Part model, mm, in its own coordinate system. Face numbers are marked on the shaded views. Give positions to 0.01 mm unless a question says otherwise; leave off trailing zeros. Write each loop counter-clockwise with the first axis right and the second up, starting at its lowest first coordinate (ties: lowest second). Pieces come first, ordered by that corner, then holes. Notation, with made-up numbers: M -4.5,57.5 L 50.5,57.5 A18 cw 50.5,91.5 Z; hole C 24,15.25 d6. An arc over 180 degrees is marked long. Answer as CSV lines item,"result". Start each with the question number.
1) Pin check, flat tips, straight feed: pin 1 Ø2 at (x, z) = (3, 7.5) entering from +Y; pin 2 Ø1 at (x, y) = (1, -22.5) entering from -Z; pin 3 Ø1.5 at (x, z) = (2, 13) entering from -Y. Stop position of each tip, or through.
2) Mould opens along Z. For the marked faces 1, 2 and 3 say: pulls with the +Z half, pulls with the -Z half, needs draft (parallel to the pull), parting line crosses it, or undercut.
3) Slice it at B-B, the plane y = -25.5. Give the cut face in (x, z).
4) Slice it at A-A, the plane x = 0.65. Give the cut face in (y, z), plus the area to 3 significant figures.
5) Wall check: line 1 along Z through (x, y) = (0.45, -21.75); line 2 along Y through (x, z) = (2.05, 10.25); line 3 along Y through (x, z) = (2.8, 10.75). Give the ranges that are in metal, low to high. Write a range as from..to.
6) Slice it at D-D, the plane x = 2.7. Give the cut face in (y, z), plus the area to 3 significant figures.
7) Slice it at C-C, the plane z = 6.25. Give the cut face in (x, y), plus the area to 3 significant figures.
```python
from build123d import *

# Parameters (mm, degrees)
SKETCH_1_R      = 5
EXTRUDE_1_DEPTH = 4
CHAMFER_1_SIZE  = 1.5
CHAMFER_1_SIZE2 = 1.616714541


with BuildPart() as part:
    # 草图1 → 凸台-拉伸1 (new body)
    with BuildSketch(Plane(origin=(0, 0, 0), x_dir=(0, 0, -1), z_dir=(1, 0, 0))):
        with Locations((-9.325362428, -21.699923803)):
            Circle(SKETCH_1_R)
    extrude(amount=EXTRUDE_1_DEPTH)

    # 切除-拉伸1 cone 1 section (through the dimple's axis) → 切除-拉伸1 (revolve, cut)
    with BuildSketch(Plane(origin=(4, -21.699923803, 9.325362428), x_dir=(0, 0, -1), z_dir=(0, 1, 0))):
        Polygon((0, 0), (1.3, 0), (0, 18.590866134), align=None)
    revolve(axis=Axis((4, -21.699923803, 9.325362428), (-1, 0, 0)), mode=Mode.SUBTRACT)

    # 倒角1
    chamfer_1_edges = [part.edges().sort_by_distance(p)[0] for p in [
        (4, -21.699923803, 10.625362428),
    ]]
    chamfer_1_side = [part.faces().sort_by_distance(p)[0] for p in [
        (4, -21.699923803, 14.183941072),
    ]]
    chamfer(chamfer_1_edges, length=CHAMFER_1_SIZE, length2=CHAMFER_1_SIZE2, reference=chamfer_1_side[0])


solid = part.part
```
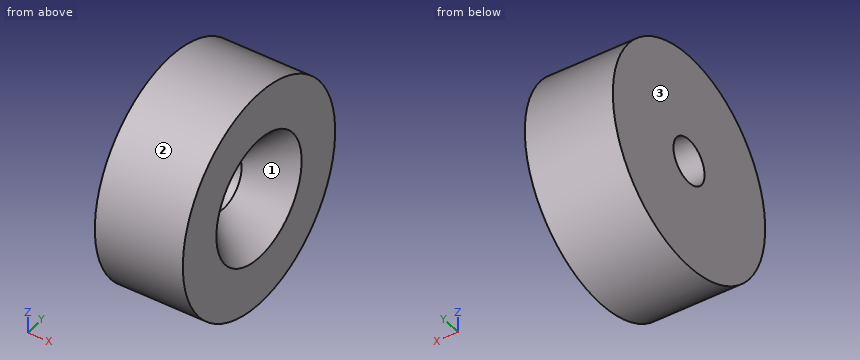
Found:
1,pin 1,"y = -16.77"
1,pin 2,"z = 4.33"
1,pin 3,"y = -25.76"
2,face 1,"undercut"
2,face 2,"parting line crosses it"
2,face 3,"needs draft"
3,outline,"M 0,6.08 L 4,6.08 L 4,12.57 L 0,12.57 Z"
4,outline,"C -21.7,9.33 d10; hole C -21.7,9.33 d2.13"
4,area,"75.0 mm²"
5,line 1,"4.33..8.27, 10.38..14.33"
5,line 2,"-26.61..-22.41, -20.99..-16.79"
5,line 3,"-26.49..-22.43, -20.97..-16.91"
6,outline,"C -21.7,9.33 d10; hole C -21.7,9.33 d3"
6,area,"71.5 mm²"
7,outline,"M 0,-25.64 L 4,-25.64 L 4,-17.76 L 0,-17.76 Z"
7,area,"31.5 mm²"
